Autodesk Inventor part; units mm, degrees
ref_plane "YZ Plane" through (0, 0, 0) normal (1, 0, 0) x (0, 1, 0)
ref_plane "XZ Plane" through (0, 0, 0) normal (0, 1, 0) x (-1, 0, 0)
ref_plane "XY Plane" through (0, 0, 0) normal (0, 0, 1) x (1, 0, 0)
sketch "Sketch1" plane through (0, 0, 0) normal (0, 1, 0) x (-1, 0, 0)
  line L0 (25, 25) -> (-25, 25)
  line L1 (-25, 25) -> (-25, -25)
  line L2 (-25, -25) -> (25, -25)
  line L3 (25, -25) -> (25, 25)
  line L4 (25, 25) -> (-25, -25) construction
  line L5 (-25, 25) -> (25, -25) construction
  point P0 (0, 0)
  dimension "d0" = 50
  dimension "d1" = 50
extrude "Extrusion1" add sketch "Sketch1" along normal blind 100
shell "Shell1" thickness 5 removed faces 1 at (8.3333, 0, -8.3333)
fillet "Fillet1" radius 19 4 edges at (0, 95, 20) (20, 95, 0) (-20, 95, 0) (0, 95, -20)
equation "\"d1\" = d0"
properties part number "traffic sign"
Model file for the job. Use its own axes, mm. A direction names the side the tool comes from. Coordinates: 2 decimals unless noted, no trailing zeros. Write each loop counter-clockwise with the first axis right and the second up, starting at its lowest first coordinate (ties: lowest second). Pieces come first, ordered by that corner, then holes. Notation, with made-up numbers: (-1, 32.5) - (52, 32.5) arc R31 ccw to (52, 59.5) - close; hole circle Ø10 at (-27, 72.5). An arc over 180 degrees is marked (long way). Write each question's results on one line, items separated by ' | '. Start each with the question number.
1) Cut at C-C (z = -15.5). Write the cut outline in (x, y).
2) 3-axis set-ups, long thin cutter, end or side, ignore diameter. For faces 1 (the face through (0, 95, 0)), 2 (the face through (-25, 49, 0)): which of +Z, -Z, +X, -X, +Y, -Y reach the whole face in a straight line?
3) Flat gauge pins, fed straight in: P1, Ø2, axis at x = -2.5, z = -17.5, coming from the -Y side; P2, Ø1, axis at x = 0, z = 0, coming from the -Y side. Where does each tip first touch, or does it go through?
4) Probe line 1 along X through (y, z) = (21.5, -8.5); line 2 along X through (y, z) = (80, -18). List the from-to ranges inside material, lowest first. Write a range as from..to.
5) Cut at D-D (y = 86). Write the cut outline in (x, z).
6) Cut at B-B (x = -9.5). Write the cut outline in (y, z).
7) Mould opens along X. For faces 3 (the face through (20, 37, 0)), 4 (the face through (23, 0, 0)), 5 (the face through (25, 49, 0)), 6 (the face through (0, 37, -20)) say: pulls with the +X half, pulls with the -X half, needs draft (parallel to the pull), parting line crosses it, or undercut.
8) Cut at A-A (y = 72.5). Write the cut outline in (x, z).
Returned:
1) outline: (-25, 0) - (-20, 0) - (-20, 76) arc R19 cw to (-15.5, 88.28) - (15.5, 88.28) arc R19 cw to (20, 76) - (20, 0) - (25, 0) - (25, 100) - (-25, 100) - close
2) face 1: -Y | face 2: +Z, -Z, -X, +Y, -Y
3) P1: y = 83.4 | P2: y = 95
4) line 1: -25..-20, 20..25 | line 2: -25..-19.57, 19.57..25
5) outline: (-25, -25) - (25, -25) - (25, 25) - (-25, 25) - close; hole (-17.16, -17.16) - (17.16, -17.16) - (17.16, 17.16) - (-17.16, 17.16) - close
6) outline: (0, -25) - (100, -25) - (100, 25) - (0, 25) - (0, 20) - (76, 20) arc R19 cw to (92.99, 9.5) - (92.99, -9.5) arc R19 cw to (76, -20) - (0, -20) - close
7) face 3: undercut | face 4: needs draft | face 5: pulls with the +X half | face 6: undercut
8) outline: (-25, -25) - (25, -25) - (25, 25) - (-25, 25) - close; hole (-20, -20) - (20, -20) - (20, 20) - (-20, 20) - close
